The listing builds one solid part. Answer for the finished solid, in the listing's coordinates (mm). A direction names the side the tool comes from. Give positions to 0.01 mm unless a question says otherwise; leave off trailing zeros. Write each loop counter-clockwise with the first axis right and the second up, starting at its lowest first coordinate (ties: lowest second). Pieces come first, ordered by that corner, then holes. Notation, with made-up numbers: (7, 31.25) - (52, 31.25) arc R9 cw to (52, 42.25) - close; hole circle Ø2 at (5.5, 80.25). An arc over 180 degrees is marked (long way). Use a Markdown table: item, result. Add a question column.
from build123d import *

# Parameters (mm, degrees)
BOSS_EXTRUDE1_DEPTH      = 10
BOSS_EXTRUDE1_DEPTH_BACK = 189.9
SKETCH1_R                = 64
SKETCH3_R                = 37.5
BOSS_EXTRUDE2_DEPTH      = 12
SKETCH4_R                = 34.103766087
CUT_EXTRUDE1_DEPTH       = 12
SKETCH5_R                = 12.5
CUT_EXTRUDE2_DEPTH       = 12
SKETCH11_R               = 12.062975476
BOSS_EXTRUDE5_DEPTH      = 42


with BuildPart() as part:
    # Sketch1 → Boss-Extrude1 (new, two sides: drawn at the far end of the back side and taken through both)
    with BuildSketch(Plane.XY.offset(-BOSS_EXTRUDE1_DEPTH_BACK)):
        Circle(SKETCH1_R)
    extrude(amount=BOSS_EXTRUDE1_DEPTH + BOSS_EXTRUDE1_DEPTH_BACK)

    # Sketch3 → Boss-Extrude2 (add)
    with BuildSketch(Plane.XY.offset(10)):
        Circle(SKETCH3_R)
    extrude(amount=BOSS_EXTRUDE2_DEPTH)

    # Sketch4 → Cut-Extrude1 (cut)
    with BuildSketch(Plane.XY.offset(22)):
        Circle(SKETCH4_R)
    extrude(amount=-CUT_EXTRUDE1_DEPTH, mode=Mode.SUBTRACT)

    # Sketch5 → Cut-Extrude2 (cut)
    with BuildSketch(Plane.XY.offset(10)):
        Circle(SKETCH5_R)
    extrude(amount=-CUT_EXTRUDE2_DEPTH, mode=Mode.SUBTRACT)

    # Sketch11 → Boss-Extrude5 (add)
    with BuildSketch(Plane.XY.offset(22)):
        with Locations(Location((17.84826857, 31.099255842, 0), (0, 0, 168.206932432))):
            Circle(SKETCH11_R)
    extrude(amount=BOSS_EXTRUDE5_DEPTH)


solid = part.part
1. The part is cut by section C-C (z = -86). Give the vertices of the cut face in (x, y).
2. For a pull along X with two mould halves and no side action, classify faces 1 (the flat face through (22, 36, 22)), 2 (the flat face through (16, 25, 22)), 3 (the cylindrical face through (22.8, 42.1, 42.7)) as released by +X, released by -X, zero draft, split by the parting line, or undercut.
3. Given P1, Ø10, axis at y = 14, z = -28, coming from the +X side; P2, Ø1, axis at x = -2.5, z = -22.5, coming from the +Y side; P3, Ø1.5, axis at x = -22, z = -124, coming from the -Y side, each flat-ended and moving along its own axis, determine where each tip first touches the part or whether it passes through.
4. The part is cut by section D-D (y = -25). Give the vertices of the cut face in (x, z).
5. Which of the six approach directions +Z, -Z, +X, -X, +Y, -Y give full straight-line access (tool end or side, diameter ignored) to faces 4 (the cylindrical face through (11.923, 3.755, 4.084)), 5 (the flat face through (18, 31, 64))?
6. Consider L1, parallel to Y at x = 0, z = 3.5; L2, parallel to Y at x = 0, z = 16; L3, parallel to Z at x = -40.5, y = -17. Determine where each line is inside the solid, lowest interval first. Write a range as [from, to].
7. The part is cut by section A-A (y = 0). Give the vertices of the cut face in (x, z), and give its area (3 significant figures).
Check values:
| question | item | result |
|---|---|---|
| 1 | outline | circle Ø128 at (0, 0) |
| 2 | face 1 | zero draft |
| 2 | face 2 | undercut |
| 2 | face 3 | split by the parting line |
| 3 | P1 | stops at x = 63.36 |
| 3 | P2 | stops at y = 63.97 |
| 3 | P3 | stops at y = -60.37 |
| 4 | outline | (-58.92, -189.9) - (58.92, -189.9) - (58.92, 10) - (27.95, 10) - (27.95, 22) - (23.2, 22) - (23.2, 10) - (-23.2, 10) - (-23.2, 22) - (-27.95, 22) - (-27.95, 10) - (-58.92, 10) - close |
| 5 | face 4 | +Z |
| 5 | face 5 | +Z, +X, -X, +Y, -Y |
| 6 | L1 | y = [-64, -12.5], [12.5, 64] |
| 6 | L2 | y = [-37.5, -34.1], [34.1, 37.5] |
| 6 | L3 | z = [-189.9, 10] |
| 7 | outline | (-64, -189.9) - (64, -189.9) - (64, 10) - (37.5, 10) - (37.5, 22) - (34.1, 22) - (34.1, 10) - (12.5, 10) - (12.5, -2) - (-12.5, -2) - (-12.5, 10) - (-34.1, 10) - (-34.1, 22) - (-37.5, 22) - (-37.5, 10) - (-64, 10) - close |
| 7 | area | 25,400 mm2 |
